```python
from build123d import *

# Parameters (mm, degrees)
SKETCH_1_W          = 18
SKETCH_1_H          = 126
EXTRUDE_1_DEPTH     = 8
SKETCH_5_W          = 13.5
SKETCH_5_H          = 55
CUT_EXTRUDE_3_DEPTH = 10
CUT_EXTRUDE_1_DEPTH = 10
FILLET_1_R          = 5
FILLET_2_R          = 5
FILLET_3_R          = 2
CUT_EXTRUDE_4_DEPTH = 8
EXTRUDE_3_DEPTH     = 8
FILLET_4_R          = 1


with BuildPart() as part:
    # 스케치1 → 보스-돌출1 (new body)
    with BuildSketch(Plane(origin=(0, 0, 0), x_dir=(1, 0, 0), z_dir=(0, 1, 0))):
        with Locations((9, 63)):
            Rectangle(SKETCH_1_W, SKETCH_1_H)
    extrude(amount=EXTRUDE_1_DEPTH)

    # 스케치5 → 컷-돌출3 (cut)
    with BuildSketch(Plane(origin=(0, 8, 0), x_dir=(1, 0, 0), z_dir=(0, 1, 0))):
        with Locations((11.25, 72.5)):
            Rectangle(SKETCH_5_W, SKETCH_5_H)
    extrude(amount=-CUT_EXTRUDE_3_DEPTH, mode=Mode.SUBTRACT)

    # 스케치2 → 컷-돌출1 (cut)
    with BuildSketch(Plane(origin=(0, 8, 0), x_dir=(1, 0, 0), z_dir=(0, 1, 0))):
        with BuildLine():
            Line((12.5, 8.25), (18, 8.25))
            ThreePointArc((18, 8.25), (21.25, 5), (18, 1.75))
            Line((18, 1.75), (12.5, 1.75))
            ThreePointArc((12.5, 1.75), (9.25, 5), (12.5, 8.25))
        make_face()
        with BuildLine():
            Line((12.5, 113.25), (18, 113.25))
            ThreePointArc((18, 113.25), (21.25, 110), (18, 106.75))
            Line((18, 106.75), (12.5, 106.75))
            ThreePointArc((12.5, 106.75), (9.25, 110), (12.5, 113.25))
        make_face()
        with BuildLine():
            Line((12.5, 38.25), (18, 38.25))
            ThreePointArc((18, 38.25), (21.25, 35), (18, 31.75))
            Line((18, 31.75), (12.5, 31.75))
            ThreePointArc((12.5, 31.75), (9.25, 35), (12.5, 38.25))
        make_face()
    extrude(amount=-CUT_EXTRUDE_1_DEPTH, mode=Mode.SUBTRACT)

    # 필렛1
    fillet_1_edges = [part.edges().sort_by_distance(p)[0] for p in [
        (4.5, 4, -45),
        (4.5, 4, -100),
    ]]
    fillet(fillet_1_edges, radius=FILLET_1_R)

    # 필렛2
    fillet_2_edges = [part.edges().sort_by_distance(p)[0] for p in [
        (18, 4, -126),
    ]]
    fillet(fillet_2_edges, radius=FILLET_2_R)

    # 필렛3
    fillet_3_edges = [part.edges().sort_by_distance(p)[0] for p in [
        (18, 4, -100),
        (18, 4, -45),
        (18, 4, -113.25),
        (18, 4, -106.75),
        (18, 4, -38.25),
        (18, 4, -31.75),
    ]]
    fillet(fillet_3_edges, radius=FILLET_3_R)

    # 스케치6 → 컷-돌출4 (cut)
    with BuildSketch(Plane.XZ):
        with BuildLine():
            Line((0, -117.5), (2.820550528, -117.5))
            ThreePointArc((2.820550528, -117.5), (3.267764124, -117.449358869), (3.692330317, -117.3))
            ThreePointArc((3.692330317, -117.3), (8, -120), (3.692330317, -122.7))
            ThreePointArc((3.692330317, -122.7), (3.267764124, -122.550641131), (2.820550528, -122.5))
            Line((2.820550528, -122.5), (0, -122.5))
            Line((0, -122.5), (0, -117.5))
        make_face()
    extrude(amount=-CUT_EXTRUDE_4_DEPTH, mode=Mode.SUBTRACT)

    # 스케치7 → 보스-돌출3 (add)
    with BuildSketch(Plane.XZ):
        with BuildLine():
            Line((9.5, 0), (9.5, 2.820550528))
            ThreePointArc((9.5, 2.820550528), (9.449358869, 3.267764124), (9.3, 3.692330317))
            ThreePointArc((9.3, 3.692330317), (12, 8), (14.7, 3.692330317))
            ThreePointArc((14.7, 3.692330317), (14.550641131, 3.267764124), (14.5, 2.820550528))
            Line((14.5, 2.820550528), (14.5, 0))
            Line((14.5, 0), (9.5, 0))
        make_face()
    extrude(amount=-EXTRUDE_3_DEPTH)

    # 필렛4
    fillet_4_edges = [part.edges().sort_by_distance(p)[0] for p in [
        (0, 4, -117.5),
        (0, 4, -122.5),
        (9.5, 4, 0),
        (14.5, 4, 0),
    ]]
    fillet(fillet_4_edges, radius=FILLET_4_R)


solid = part.part
```
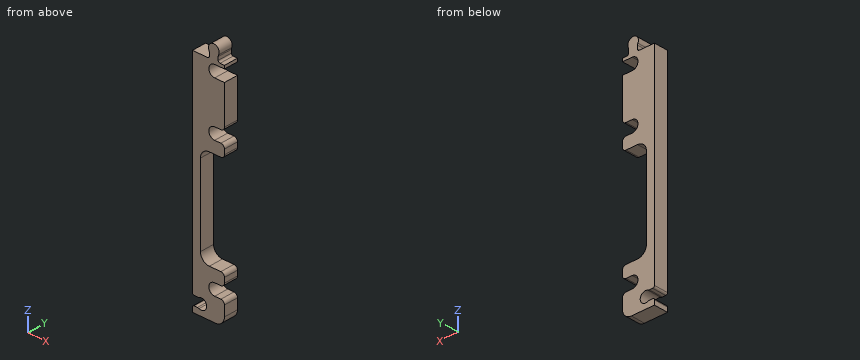
CAD build for the part. Positions are in the model's coordinates, mm. Round coordinates to 2 decimals unless told otherwise and drop trailing zeros. Order: outer loops, then holes, each group sorted by start corner. A loop starts at its lowest first (then second) coordinate and runs counter-clockwise, first axis right, second up. Notation, with made-up numbers: (-28, -34.75) - (5, -34.75) arc R19 cw to (5, -2.75) - close; hole circle Ø9 at (-13.5, 45.5). An arc over 180 degrees is marked (long way). Answer in a Markdown table with one row per item. Add a question column.
(1) Band-saw the part on C-C on z = -110. List the corners of the cut face in (x, y), and give its area (3 significant figures).
(2) Band-saw the part on B-B on z = 5. List the corners of the cut face in (x, y).
(3) Probe L1, parallel to Z at x = 12, y = 4.5; L2, parallel to Z at x = 16, y = 1; L3, parallel to Z at x = 5, y = 5.5. List the from-to ranges inside material, lowest first. Write a range as [from, to].
(4) Drop flat-ended pins along their axis: pin 1 Ø2 at (y, z) = (5.5, 1.5) entering from -X; pin 2 Ø3 at (y, z) = (2.5, -64) entering from +X; pin 3 Ø1 at (x, y) = (15, 5.5) entering from +Z. Give the stop position or say it passes through.
(5) Band-saw the part on A-A on x = 6.5. List the corners of the cut face in (y, z).
Data:
| question | item | result |
|---|---|---|
| 1 | outline | (0, 0) - (9.25, 0) - (9.25, 8) - (0, 8) - close |
| 1 | area | 74.0 mm^2 |
| 2 | outline | (9, 0) - (15, 0) - (15, 8) - (9, 8) - close |
| 3 | L1 | z = [-126, -113.21], [-106.79, -100], [-45, -38.21], [-31.79, -8.21], [-1.79, 8] |
| 3 | L2 | z = [-125, -113.25], [-106.75, -100], [-45, -38.25], [-31.75, -8.25], [-1.75, 0] |
| 3 | L3 | z = [-126, -123], [-117, -97.18], [-47.82, 0] |
| 4 | pin 1 | stops at x = 9.37 |
| 4 | pin 2 | stops at x = 4.5 |
| 4 | pin 3 | stops at z = 6.66 |
| 5 | outline | (0, -126) - (8, -126) - (8, -122.6) - (0, -122.6) - close; (0, -117.4) - (8, -117.4) - (8, -99) - (0, -99) - close; (0, -46) - (8, -46) - (8, 0) - (0, 0) - close |
